from build123d import *

# Parameters (mm, degrees)
BOSS_EXTRUDE2_DEPTH      = 63.5
BOSS_EXTRUDE2_DEPTH_BACK = 0.000100076
FILLET2_R                = 2.54


with BuildPart() as part:
    # Sketch2 → Boss-Extrude2 (new, two sides: drawn at the far end of the back side and taken through both)
    with BuildSketch(Plane(origin=(0, 0, 0), x_dir=(1, 0, 0), z_dir=(0, 1, 0)).offset(-BOSS_EXTRUDE2_DEPTH_BACK)):
        Polygon((7.336319495, 7.83629969), (7.336319495, 0), (29.508870684, 0), align=None)
        Polygon((29.508870684, 0), (7.336319495, 0), (7.336319495, -7.83629969), align=None)
        Polygon((7.336319495, 0), (-3.449421721, 0), (-0.116444388, -10.257849467), (7.336319495, -7.83629969), align=None)
        Polygon((-0.116444388, 10.257849467), (-3.449421721, 0), (7.336319495, 0), (7.336319495, 7.83629969), align=None)
        Polygon((-12.175269662, 6.339699622), (-3.449421721, 0), (-0.116444388, 10.257849467), (-7.569208272, 12.679399244), align=None)
        Polygon((-12.175269662, -6.339699622), (-3.449421721, 0), (-12.175269662, 6.339699622), (-16.781331052, 0), align=None)
        Polygon((-0.116444388, -10.257849467), (-3.449421721, 0), (-12.175269662, -6.339699622), (-7.569208272, -12.679399244), align=None)
        Polygon((6.735250738, -31.345198758), (-0.116444388, -10.257849467), (-7.569208272, -12.679399244), align=None)
        Polygon((7.336319495, -7.83629969), (-0.116444388, -10.257849467), (6.735250738, -31.345198758), align=None)
        Polygon((-7.569208272, -12.679399244), (-12.175269662, -6.339699622), (-30.113240383, -19.372398217), align=None)
        Polygon((-30.113240383, -19.372398217), (-12.175269662, -6.339699622), (-16.781331052, 0), align=None)
        Polygon((-16.781331052, 0), (-12.175269662, 6.339699622), (-30.113240383, 19.372398217), align=None)
        Polygon((-30.113240383, 19.372398217), (-12.175269662, 6.339699622), (-7.569208272, 12.679399244), align=None)
        Polygon((-7.569208272, 12.679399244), (-0.116444388, 10.257849467), (6.735250738, 31.345198758), align=None)
        Polygon((6.735250738, 31.345198758), (-0.116444388, 10.257849467), (7.336319495, 7.83629969), align=None)
    extrude(amount=BOSS_EXTRUDE2_DEPTH + BOSS_EXTRUDE2_DEPTH_BACK)

    # Fillet2
    fillet2_edges = [part.edges().sort_by_distance(p)[0] for p in [
        (-16.781331052, 31.749949962, 0),
        (-30.113240383, 31.749949962, -19.372398217),
        (-7.569208272, 31.749949962, -12.679399244),
        (6.735250738, 31.749949962, -31.345198758),
        (7.336319495, 31.749949962, -7.83629969),
        (29.508870684, 31.749949962, 0),
        (7.336319495, 31.749949962, 7.83629969),
        (6.735250738, 31.749949962, 31.345198758),
        (-7.569208272, 31.749949962, 12.679399244),
        (-30.113240383, 31.749949962, 19.372398217),
    ]]
    fillet(fillet2_edges, radius=FILLET2_R)


solid = part.part
Input: part model. Units: mm. Frame: model coordinates. A direction names the side the tool comes from. Give positions to 0.01 mm unless a question says otherwise; leave off trailing zeros. Loops run counter-clockwise (first coordinate to the right, second up) from the corner with the lowest first, then second, coordinate; pieces in that order, holes last. Notation, with made-up numbers: (80.25, 87.5) - (118.25, 87.5) arc R12 cw to (118.25, 91.5) - close; hole circle Ø5 at (69, 85.25). An arc over 180 degrees is marked (long way). Use CSV: the item, a comma, the result in double quotes. Start each with the question number.
Item 1: Mould query, pull axis X, two halves, no side actions, for faces 1 (the cylindrical face through (5.123, 32.194, 26.525)), 2 (the cylindrical face through (-7.72, 32.19, -13.2)), 3 (the cylindrical face through (7.789, 32.194, -8.138)). Classes: pulls with the +X half, pulls with the -X half, needs draft (parallel to the pull), parting line crosses it, or undercut.
Item 2: Section D-D on x = 10. Return loops of the section in (y, z), then the cut area to 3 significant figures.
Item 3: Section C-C on z = 22. Return loops of the section in (x, y), then the cut area to 3 significant figures.
Item 4: Contact query for flat-ended pins moving along their axis: P1, Ø4, axis at x = 8.5, y = 7.5, coming from the +Z side; P2, Ø6, axis at x = 9.5, y = 36, coming from the -Z side; P3, Ø1, axis at x = -1, y = 38.5, coming from the +Z side. Output: stop coordinate, or through.
Item 5: Reachability of faces 4 (the flat face through (-2.133, 31.305, 19.773)), 5 (the cylindrical face through (-17.325, 32.194, -0.021)), 6 (the flat face through (-16.136, 31.305, -15.223)) from +Z, -Z, +X, -X, +Y, -Y: full face, straight path, thin tool, end or side. Return the list, or none.
Item 6: Section B-B on y = 26. Return loops of the section in (x, z), then the cut area to 3 significant figures.
Item 7: Section A-A on x = -22. Return loops of the section in (y, z).
Item 8: Line query: line 1 (Z direction, x = -19, y = 11); line 2 (X direction, y = 48, z = 0); line 3 (Z direction, x = -13, y = 15). Output: solid intervals per line, ascending.
Ans:
1,face 1,"parting line crosses it"
1,face 2,"undercut"
1,face 3,"pulls with the +X half"
2,outline,"(0, -6.89) - (63.5, -6.89) - (63.5, 6.89) - (0, 6.89) - close"
2,area,"876 mm2"
3,outline,"(-0.43, 0) - (6.97, 0) - (6.97, 63.5) - (-0.43, 63.5) - close"
3,area,"470 mm2"
4,P1,"stops at z = 25.49"
4,P2,"stops at z = -25.49"
4,P3,"stops at z = 21.9"
5,face 4,"+Z, +Y, -Y"
5,face 5,"-X, +Y, -Y"
5,face 6,"-Z, +Y, -Y"
6,outline,"(-26.04, -13.45) arc R2.54 ccw to (-23.22, -17.33) - (-9.24, -13.18) arc R2.54 cw to (-6.51, -14.07) - (2.36, -25.64) arc R2.54 ccw to (6.92, -24.16) - (7.29, -9.58) arc R2.54 cw to (8.98, -7.25) - (22.73, -2.39) arc R2.54 ccw to (22.73, 2.39) - (8.98, 7.25) arc R2.54 cw to (7.29, 9.58) - (6.92, 24.16) arc R2.54 ccw to (2.36, 25.64) - (-6.51, 14.07) arc R2.54 cw to (-9.24, 13.18) - (-23.22, 17.33) arc R2.54 ccw to (-26.04, 13.45) - (-17.77, 1.44) arc R2.54 cw to (-17.77, -1.44) - close"
6,area,"1,240 mm2"
7,outline,"(0, -16.96) - (63.5, -16.96) - (63.5, -7.58) - (0, -7.58) - close; (0, 7.58) - (63.5, 7.58) - (63.5, 16.96) - (0, 16.96) - close"
8,line 1,"z = -16.07 to -3.22, 3.22 to 16.07"
8,line 2,"x = -17.32 to 24.43"
8,line 3,"z = -14.29 to 14.29"
